from build123d import *

# Parameters (mm, degrees)
F0_R     = 6.375
F1_DEPTH = 21
F0_R_2   = 65
F0_R_3   = 12.5
F0_R_4   = 13.2
F0_R_5   = 12
F0_R_6   = 11.1
F0_R_7   = 14.1
F0_R_8   = 14.45
F0_R_9   = 10.4
F0_R_10  = 9.25
F2_DEPTH = 15
F3_T     = 2.5


with BuildPart() as f1:
    # F0 (on Top) → F1 (new body)
    with BuildSketch(Plane.XY):
        Circle(F0_R)
    extrude(amount=F1_DEPTH)

    # F0 (on Top) → F2 (join)
    with BuildSketch(Plane.XY):
        Circle(F0_R_2)
        with Locations((-16.245956808, -44.6353994873)):
            Circle(F0_R_3, mode=Mode.SUBTRACT)
        with Locations((-41.1362066798, -23.75)):
            Circle(F0_R_4, mode=Mode.SUBTRACT)
        with Locations((16.245956808, -44.6353994873)):
            Circle(F0_R_5, mode=Mode.SUBTRACT)
        with Locations((41.1362066798, -23.75)):
            Circle(F0_R_6, mode=Mode.SUBTRACT)
        with Locations((-46.7783682681, 8.2482884392)):
            Circle(F0_R_7, mode=Mode.SUBTRACT)
        with Locations((-30.5324114601, 36.3871110482)):
            Circle(F0_R_8, mode=Mode.SUBTRACT)
        Circle(F0_R, mode=Mode.SUBTRACT)
        with Locations((46.7783682681, 8.2482884392)):
            Circle(F0_R_9, mode=Mode.SUBTRACT)
        with Locations((30.5324114601, 36.3871110482)):
            Circle(F0_R_10, mode=Mode.SUBTRACT)
    extrude(amount=F2_DEPTH)

    # F3
    f3_openings = [f1.faces().sort_by_distance(p)[0] for p in [
        (3.404358, 2.387056, 0),
    ]]
    offset(amount=F3_T, openings=f3_openings, kind=Kind.INTERSECTION)


solid = f1.part
Here's how the part is built. I have some questions about the finished solid (model axes, mm). A direction names the side the tool comes from. Coordinates: 2 decimals unless noted, no trailing zeros. Order: outer loops, then holes, each group sorted by start corner. A loop starts at its lowest first (then second) coordinate and runs counter-clockwise, first axis right, second up.
Item 1: If we section it at A-A on z = 11.25: State how many separate pieces and enclosed holes the cut face has, plus the area to 3 significant figures.
Result sheet:
separate pieces: 9
enclosed holes: 9
area: 2,410 mm2
Item 2: I need wall thicknesses on line 1 (X direction, y = 1, z = 6.25); line 2 (Y direction, x = 18.5, z = 3.5); line 3 (Y direction, x = -29.5, z = 3.5). Which ranges of each line are inside material? Lowest first, please.
Result sheet:
line 1: x = -67.49 to -64.99, -58.87 to -55.83, -37.72 to -34.68, 39.32 to 43.64, 49.92 to 54.24, 64.99 to 67.49
line 2: y = -64.92 to -62.31, -56.42 to -53.86, -35.41 to -32.85, 62.31 to 64.92
line 3: y = -60.71 to -57.92, -29.98 to -17.52, 21.97 to 24.48, 48.29 to 50.8, 57.92 to 60.71
Item 3: If we section it at C-C on x = -49: List the corners of the cut face in (y, z) for me, plus the area to 3 significant figures.
Result sheet:
outline: (-46.42, 0) - (-42.71, 0) - (-42.71, 15) - (-34.35, 15) - (-34.35, 0) - (-31.01, 0) - (-31.01, 17.5) - (-46.42, 17.5) - close; (-16.49, 0) - (-13.15, 0) - (-13.15, 15) - (-5.68, 15) - (-5.68, 0) - (-3.14, 0) - (-3.14, 17.5) - (-16.49, 17.5) - close; (19.63, 0) - (22.17, 0) - (22.17, 15) - (42.71, 15) - (42.71, 0) - (46.42, 0) - (46.42, 17.5) - (19.63, 17.5) - close
area: 427 mm2
Item 4: For P1, Ø4, axis at y = 38, z = 15.5, coming from the +X side; P2, Ø14, axis at x = 1.5, y = -2.5, coming from the -Z side; P3, Ø5, axis at x = 16.5, z = 5.5, coming from the +Y side; P4, Ø10, axis at x = -27, y = 38, coming from the +Z side, each with a flat end and sliding along its axis, tell me the tip position at first contact or that it passes through.
Result sheet:
P1: stops at x = 57.1
P2: stops at z = 15
P3: stops at y = 66.03
P4: passes through
Item 5: If we mould it in two halves opening along Y, with no side actions, what happens to faces 3 (the face through (-44.97, 37.02, 7.4)), 4 (the face through (-41.2, -12.9, 0)), 5 (the face through (-1.924, -8.664, 20.458))? For each: +Y half, -Y half, draft (parallel to the pull), parting line (faces both ways), or undercut.
Result sheet:
face 3: undercut
face 4: draft
face 5: parting line
Item 6: For faces 1 (the face through (-28.943, -28.806, 7.395)), 2 (the face through (-31.252, -27.848, 8.628)), which set-ups out of +Z, -Z, +X, -X, +Y, -Y let a thin tool reach every point of the face, with its end or its side?
Result sheet:
face 1: -Z
face 2: +Z, -Z
Item 7: If we section it at B-B on y = -23.75: List the corners of the cut face in (x, z) for me.
Result sheet:
outline: (-63.18, 0) - (-60.51, 0) - (-60.51, 15) - (-54.34, 15) - (-54.34, 0) - (-51.84, 0) - (-51.84, 17.5) - (-63.18, 17.5) - close; (-30.44, 0) - (-27.94, 0) - (-27.94, 15) - (30.04, 15) - (30.04, 0) - (32.54, 0) - (32.54, 17.5) - (-30.44, 17.5) - close; (49.74, 0) - (52.24, 0) - (52.24, 15) - (60.51, 15) - (60.51, 0) - (63.18, 0) - (63.18, 17.5) - (49.74, 17.5) - close
